Could you check a few things on this model? Use its own coordinates, in mm. Give positions to 0.01 mm unless a question says otherwise; leave off trailing zeros. Order: outer loops, then holes, each group sorted by start corner. A loop starts at its lowest first (then second) coordinate and runs counter-clockwise, first axis right, second up. Notation, with made-up numbers: (-26, 48) -> (-2, 48) arc R18 cw to (-2, 82) -> close; hole circle Ø2 at (66.25, 55). An arc over 180 degrees is marked (long way). Answer as CSV lines item,"result". Start each with the question number.
(1) Will these pins go through, and if not, where does the flat tip stop? pin 1 Ø1.6 at (x, y) = (-32.5, 10.25) entering from -Z; pin 2 Ø2.5 at (x, y) = (-32.5, -10.25) entering from +Z.
(2) I need wall thicknesses on L1, parallel to Y at x = -32.5, z = 0.15; L2, parallel to X at y = -10.25, z = 0.1; L3, parallel to X at y = -3.5, z = 0.3. Which ranges of each line are inside material? Lowest first, please.
(3) I want a section at D-D (x = 13.5). Please give me the cut outline in (y, z), plus the area to 3 significant figures.
(4) I want a section at C-C (y = -0.75). Please give me the cut outline in (x, z), plus the area to 3 significant figures.
(5) I want a section at A-A (x = -7.5). Please give me the cut outline in (y, z).
(6) I want a section at B-B (z = 0.4). Give the number of separate pieces and of enclosed holes in the cut face, plus the area to 3 significant figures.
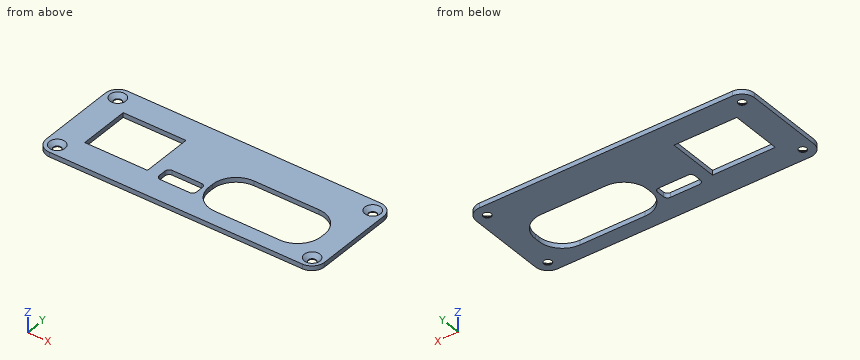
Autodesk Inventor part; units mm, degrees
ref_plane "YZ Plane" through (0, 0, 0) normal (1, 0, 0) x (0, 1, 0)
ref_plane "XZ Plane" through (0, 0, 0) normal (0, 1, 0) x (-1, 0, 0)
ref_plane "XY Plane" through (0, 0, 0) normal (0, 0, 1) x (1, 0, 0)
sketch "Sketch1" plane through (0, 0, 0) normal (0, 0, 1) x (1, 0, 0)
  line L0 (-35.5, 13.25) -> (35.5, 13.25)
  line L1 (35.5, 13.25) -> (35.5, -13.25)
  line L2 (35.5, -13.25) -> (-35.5, -13.25)
  line L3 (-35.5, -13.25) -> (-35.5, 13.25)
  point P0 (0, 0)
  dimension "d0" = 26.5
  dimension "d1" = 71
  dimension "d2" = 35.5
  dimension "d3" = 13.25
extrude "Extrusion1" add sketch "Sketch1" along normal blind 1.2
fillet "Fillet1" radius 3.25 4 edges at (-35.5, 13.25, 0.6) (-35.5, -13.25, 0.6) (35.5, -13.25, 0.6) (35.5, 13.25, 0.6)
sketch "Sketch2" plane through (0, 0, 1.2) normal (0, 0, 1) x (1, 0, 0)
  line L0 (32.25, 13.25) -> (-32.25, 13.25)
  line L1 (-35.5, 10) -> (-35.5, -10)
  line L2 (-32.25, -13.25) -> (32.25, -13.25)
  line L3 (35.5, -10) -> (35.5, 10)
  point P0 (0, 0)
  point P1 (-32.5, 10.25)
  point P2 (32.5, 10.25)
  point P3 (32.5, -10.25)
  point P4 (-32.5, -10.25)
  dimension "d7" = 3
  dimension "d8" = 3
  dimension "d9" = 3
  dimension "d10" = 3
  dimension "d11" = 3
  dimension "d12" = 3
  dimension "d13" = 3
  dimension "d14" = 3
hole "Hole1" at (-32.5, 10.25, 1.2) at (32.5, 10.25, 1.2) at (32.5, -10.25, 1.2) at (-32.5, -10.25, 1.2) direction (0, 0, -1) diameter 2 depth 4 tip angle 118 countersink diameter 4 countersink angle 90
sketch "Sketch3" plane through (0, 0, 1.2) normal (0, 0, 1) x (1, 0, 0)
  line L0 (-28.5, 6.75) -> (-12.5, 6.75)
  line L1 (-12.5, 6.75) -> (-12.5, -6.25)
  line L2 (-12.5, -6.25) -> (-28.5, -6.25)
  line L3 (-28.5, -6.25) -> (-28.5, 6.75)
  line L4 (-35.5, 10) -> (-35.5, -10)
  line L5 (-32.25, -13.25) -> (32.25, -13.25)
  point P0 (0, 0)
  dimension "d22" = 7
  dimension "d23" = 23
  dimension "d24" = 7
  dimension "d25" = 20
extrude "Extrusion2" cut sketch "Sketch3" against normal blind 2
sketch "Sketch4" plane through (0, 0, 1.2) normal (0, 0, 1) x (1, 0, 0)
  line L0 (-9.5, -3.25) -> (0, -3.25)
  line L1 (0, -3.25) -> (0, -7.25)
  line L2 (0, -7.25) -> (-9.5, -7.25)
  line L3 (-9.5, -7.25) -> (-9.5, -3.25)
  line L4 (-35.5, 10) -> (-35.5, -10)
  line L5 (-32.25, -13.25) -> (32.25, -13.25)
  point P0 (0, 0)
  dimension "d28" = 26
  dimension "d29" = 35.5
  dimension "d30" = 6
  dimension "d31" = 10
extrude "Extrusion3" cut sketch "Sketch4" against normal blind 2
sketch "Sketch5" plane through (0, 0, 1.2) normal (0, 0, 1) x (1, 0, 0)
  line L0 (6.5, 1.75) -> (24.5, 1.75)
  line L1 (24.5, 1.75) -> (24.5, -5.25)
  line L2 (24.5, -5.25) -> (6.5, -5.25)
  line L3 (6.5, -5.25) -> (6.5, 1.75)
  line L4 (35.5, -10) -> (35.5, 10)
  line L5 (-32.25, -13.25) -> (32.25, -13.25)
  point P0 (0, 0)
  dimension "d34" = 11
  dimension "d35" = 29
  dimension "d36" = 15
  dimension "d37" = 8
extrude "Extrusion4" cut sketch "Sketch5" against normal blind 2
chamfer "Chamfer1" distance 2 angle 45 2 edges at (6.5, -5.25, 0.6) (24.5, -5.25, 0.6)
fillet "Fillet2" radius 1 4 edges at (-9.5, -3.25, 0.6) (-9.5, -7.25, 0.6) (0, -7.25, 0.6) (0, -3.25, 0.6)
sketch "Sketch7" plane through (0, 0, 1.2) normal (0, 0, 1) x (1, 0, 0)
  line L0 (1, 3.85) -> (29.6, 3.85)
  line L1 (29.6, 3.85) -> (29.6, -9.35)
  line L2 (29.6, -9.35) -> (1, -9.35)
  line L3 (1, -9.35) -> (1, 3.85)
  line L4 (-32.25, -13.25) -> (32.25, -13.25)
  line L5 (35.5, -10) -> (35.5, 10)
  point P0 (0, 0)
  dimension "d56" = 3.9
  dimension "d57" = 5.9
  dimension "d58" = 17.1
  dimension "d59" = 34.5
extrude "Extrusion6" cut sketch "Sketch7" against normal blind 2
fillet "Fillet3" radius 6 4 edges at (1, 3.85, 0.6) (1, -9.35, 0.6) (29.6, 3.85, 0.6) (29.6, -9.35, 0.6)
properties part number "cover-slave"
Final values:
1,pin 1,"through"
1,pin 2,"z = 0.45"
2,L1,"-13.24 to -11.25, -9.25 to 9.25, 11.25 to 13.24"
2,L2,"-35.49 to -33.5, -31.5 to 31.5, 33.5 to 35.49"
2,L3,"-35.5 to -28.5, -12.5 to -9.16, -0.34 to 1, 29.6 to 35.5"
3,outline,"(-13.25, 0) -> (-9.35, 0) -> (-9.35, 1.2) -> (-13.25, 1.2) -> close; (3.85, 0) -> (13.25, 0) -> (13.25, 1.2) -> (3.85, 1.2) -> close"
3,area,"16.0 mm²"
4,outline,"(-35.5, 0) -> (-28.5, 0) -> (-28.5, 1.2) -> (-35.5, 1.2) -> close; (-12.5, 0) -> (1.17, 0) -> (1.17, 1.2) -> (-12.5, 1.2) -> close; (29.43, 0) -> (35.5, 0) -> (35.5, 1.2) -> (29.43, 1.2) -> close"
4,area,"32.1 mm²"
5,outline,"(-13.25, 0) -> (-7.25, 0) -> (-7.25, 1.2) -> (-13.25, 1.2) -> close; (-3.25, 0) -> (13.25, 0) -> (13.25, 1.2) -> (-3.25, 1.2) -> close"
6,separate pieces,"1"
6,enclosed holes,"7"
6,area,"1,260 mm²"
